from build123d import *

# Parameters (mm, degrees)
SKETCH_R        = 6
PAD_DEPTH       = 4
SKETCH001_R     = 6.47535
PAD001_DEPTH    = 1
SKETCH002_R     = 6
PAD002_DEPTH    = 4
SKETCH003_R     = 4
POCKET_DEPTH    = 9.001
PAD003_DEPTH    = 4
SKETCH005_R     = 1.55
POCKET001_DEPTH = 9.001


with BuildPart() as part:
    # Sketch → Pad (new body)
    with BuildSketch(Plane.XY):
        with Locations((0.5, 0)):
            Circle(SKETCH_R)
    extrude(amount=-PAD_DEPTH)

    # Sketch001 (on Face3 of Pad) → Pad001 (join)
    with BuildSketch(Plane(origin=(0, 0, -4), x_dir=(1, 0, 0), z_dir=(0, 0, -1))):
        Circle(SKETCH001_R)
    extrude(amount=PAD001_DEPTH)

    # Sketch002 (on Face6 of Pad001) → Pad002 (join)
    with BuildSketch(Plane(origin=(0, 0, -5), x_dir=(1, 0, 0), z_dir=(0, 0, -1))):
        with Locations((-0.5, 0)):
            Circle(SKETCH002_R)
    extrude(amount=PAD002_DEPTH)

    # Sketch003 (on Face2 of Pad002) → Pocket (cut, through all)
    with BuildSketch(Plane.XY):
        Circle(SKETCH003_R)
    extrude(amount=-POCKET_DEPTH, mode=Mode.SUBTRACT)

    # Sketch004 (on Face7 of Pocket) → Pad003 (join)
    with BuildSketch(Plane(origin=(0, 0, -9), x_dir=(1, 0, 0), z_dir=(0, 0, -1))):
        with BuildLine():
            ThreePointArc((-3, 2.645751), (-4, 0), (-3, -2.645751))
            Line((-3, 2.645751), (-3, -2.645751))
        make_face()
    extrude(amount=-PAD003_DEPTH)

    # Sketch005 (on Face7 of Pad003) → Pocket001 (cut, through all)
    with BuildSketch(Plane(origin=(0, 0, -9), x_dir=(1, 0, 0), z_dir=(0, 0, -1))):
        with Locations((-1.65, 2)):
            Circle(SKETCH005_R)
        with Locations((-1.65, -2)):
            Circle(SKETCH005_R)
    extrude(amount=-POCKET001_DEPTH, mode=Mode.SUBTRACT)


solid = part.part
Geometry check sheet. Reference: the model listing, model coordinates, mm. A direction names the side the tool comes from. Round coordinates to 2 decimals unless told otherwise and drop trailing zeros. Order: outer loops, then holes, each group sorted by start corner. A loop starts at its lowest first (then second) coordinate and runs counter-clockwise, first axis right, second up. Notation, with made-up numbers: M 30.5,16.25 L 66.5,16.25 A18 ccw 66.5,36.25 Z; hole C -32,29 d9. An arc over 180 degrees is marked long. Answer in a Markdown table with one row per item. Add a question column.
Item 1: Sectioned sample at D-D, the plane y = -5.25. Enter the section's corners in (x, z).
Item 2: Sectioned sample at C-C, the plane x = 0. Enter the section's corners in (y, z), plus the area to 3 significant figures.
Item 3: Material ranges on L1, parallel to Y at x = 0, z = -4.75; L2, parallel to X at y = 0, z = -5.75; L3, parallel to Z at x = -4, y = 5, recorded low to high. Write a range as [from, to].
Item 4: Set-up check for faces 4 (the face through (-3.5, 0, -5)), 5 (the face through (-3, 0, -7)), 6 (the face through (-5.26, 3.65, -6.97)): record each of +Z, -Z, +X, -X, +Y, -Y from which the full face is reachable in a straight line by a thin tool's end or side.
Item 5: Draft check along X on faces 1 (the face through (-4.26, -3.65, -1.97)), 2 (the face through (-6, 0, -4)), 3 (the face through (-4, 0, -2)). Enter one of: released by +X, released by -X, zero draft, split by the parting line, or undercut.
Item 6: Depth check by flat-ended pin: pin 1 Ø5 at (x, z) = (5, -3.5) entering from -Y; pin 2 Ø1.2 at (y, z) = (-0.5, -6) entering from +X. Enter the tip coordinate at first touch or a pass-through.
Item 7: Sectioned sample at A-A, the plane z = -8.5. Enter the section's corners in (x, y), plus the area to 3 significant figures.
Filled in:
| question | item | result |
|---|---|---|
| 1 | outline | M -3.79,-5 L -3.4,-5 L -3.4,-9 L 2.4,-9 L 2.4,-5 L 3.79,-5 L 3.79,-4 L 3.4,-4 L 3.4,0 L -2.4,0 L -2.4,-4 L -3.79,-4 Z |
| 2 | outline | M -6.48,-5 L -5.98,-5 L -5.98,-9 L -4,-9 L -4,0 L -5.98,0 L -5.98,-4 L -6.48,-4 Z; M 4,-9 L 5.98,-9 L 5.98,-5 L 6.48,-5 L 6.48,-4 L 5.98,-4 L 5.98,0 L 4,0 Z |
| 2 | area | 36.6 mm² |
| 3 | L1 | y = [-6.48, -4], [4, 6.48] |
| 3 | L2 | x = [-6.5, -3], [4, 5.5] |
| 3 | L3 | z = [-5, -4] |
| 4 | face 4 | +Z |
| 4 | face 5 | +Z, -Z |
| 4 | face 6 | -Z |
| 5 | face 1 | split by the parting line |
| 5 | face 2 | zero draft |
| 5 | face 3 | undercut |
| 6 | pin 1 | stops at y = -5.95 |
| 6 | pin 2 | stops at x = 5.5 |
| 7 | outline | C -0.5,0 d12; hole M -3,-1.24 A1.55 ccw -1.87,-3.53 A4 ccw long -1.87,3.53 A1.55 ccw -3,1.24 Z |
| 7 | area | 65.7 mm² |
